from build123d import *

# Parameters (mm, degrees)
F1_DEPTH = 103.378
F2_T     = -2.54


with BuildPart() as f1:
    # F0 (on Front) → F1 (new body)
    with BuildSketch(Plane.XZ):
        Polygon((-71.7586703687, 0), (0, 0), (40.1820645289, 0), (40.1820645289, 119.9224553038), (-27.8168563806, 44.4326761603), (-71.7586703687, 94.0080558437), align=None)
    extrude(amount=F1_DEPTH)

    # F2
    f2_openings = [f1.faces().sort_by_distance(p)[0] for p in [
        (-15.788303, -51.689, 0),
    ]]
    offset(amount=F2_T, openings=f2_openings, kind=Kind.INTERSECTION)


solid = f1.part
Design review of the part built by this model. Coordinates are the model's own, in mm. A direction names the side the tool comes from. Round coordinates to 2 decimals unless told otherwise and drop trailing zeros. Order: outer loops, then holes, each group sorted by start corner. A loop starts at its lowest first (then second) coordinate and runs counter-clockwise, first axis right, second up. Notation, with made-up numbers: M 33,-34.5 L 53,-34.5 A11 ccw 53,-29.5 Z; hole C 0.5,-8 d8. An arc over 180 degrees is marked long. Answer as CSV lines item,"result". Start each with the question number.
1) Add section D-D (x = 29). Give the boundary of the cut face in (y, z), then the cut area to 3 significant figures.
2) Add section A-A (z = 82). Give the boundary of the cut face in (x, y), then the cut area to 3 significant figures.
3) Wall thickness on line 1 along X through (y, z) = (-92.5, 6); line 2 along Y through (x, z) = (-7.5, 26); line 3 along X through (y, z) = (-82, 76): over which ranges is each line inside the solid? List them lowest first. Write a range as [from, to].
4) Tool access review of faces 5 (the face through (-49.48, -50.965, 68.873)), 6 (the face through (-20, -101, 0)), 7 (the face through (37.642, -51, 56)): name each direction out of +Z, -Z, +X, -X, +Y, -Y from which nothing blocks a thin tool from reaching the whole face with its end or side.
5) For pin 1 Ø1.5 at (x, y) = (-11.5, -35.5) entering from +Z; pin 2 Ø10 at (x, z) = (1.5, 87) entering from -Y; pin 3 Ø1.5 at (x, y) = (-55, -30.5) entering from +Z; pin 4 Ø8 at (x, y) = (-56.5, -77.5) entering from +Z, all flat-tipped, find the tip position at first contact; note any pin that passes through.
6) The part is to be moulded in two halves that separate along X. For faces 1 (the face through (-17, -103.378, 34)), 2 (the face through (-17, -100.838, 32)), 3 (the face through (-71.759, -51, 48)), 4 (the face through (6.66, -50.97, 82.71)), say which applies: +X half, -X half, draft (parallel to the pull), parting line (faces both ways), or undercut.
7) Add section B-B (y = -36.5). Give the boundary of the cut face in (x, z), then the cut area to 3 significant figures.
8) Add section C-C (z = 105). Give the boundary of the cut face in (x, y), then the cut area to 3 significant figures.
Resolved:
1,outline,"M -103.38,0 L -100.84,0 L -100.84,103.71 L -2.54,103.71 L -2.54,0 L 0,0 L 0,107.51 L -103.38,107.51 Z"
1,area,"919 mm^2"
2,outline,"M -71.76,-103.38 L -61.12,-103.38 L -61.12,0 L -71.76,0 Z; M 6.02,-103.38 L 40.18,-103.38 L 40.18,0 L 6.02,0 Z; hole M -69.22,-100.84 L -64.51,-100.84 L -64.51,-2.54 L -69.22,-2.54 Z; hole M 9.44,-100.84 L 37.64,-100.84 L 37.64,-2.54 L 9.44,-2.54 Z"
2,area,"1,400 mm^2"
3,line 1,"[-71.76, -69.22], [37.64, 40.18]"
3,line 2,"[-103.38, -100.84], [-2.54, 0]"
3,line 3,"[-71.76, -69.22], [-59.19, -55.8], [0.62, 4.04], [37.64, 40.18]"
4,face 5,"+Z, +Y, -Y"
4,face 6,"-Z, +X, -X, +Y, -Y"
4,face 7,"-Z"
5,pin 1,"z = 63.38"
5,pin 2,"through"
5,pin 3,"z = 75.95"
5,pin 4,"z = 81.31"
6,face 1,"draft"
6,face 2,"undercut"
6,face 3,"-X half"
6,face 4,"undercut"
7,outline,"M -71.76,0 L -69.22,0 L -69.22,87.31 L -27.83,40.62 L 37.64,113.31 L 37.64,0 L 40.18,0 L 40.18,119.92 L -27.82,44.43 L -71.76,94.01 Z"
7,area,"943 mm^2"
8,outline,"M 26.74,-103.38 L 40.18,-103.38 L 40.18,0 L 26.74,0 Z; hole M 30.16,-100.84 L 37.64,-100.84 L 37.64,-2.54 L 30.16,-2.54 Z"
8,area,"654 mm^2"
